Can you work these out from the model? Positions are in its coordinate system, mm. Face numbers are marked on the shaded views. A direction names the side the tool comes from. Coordinates: 2 decimals unless noted, no trailing zeros. Loops run counter-clockwise (first coordinate to the right, second up) from the corner with the lowest first, then second, coordinate; pieces in that order, holes last.
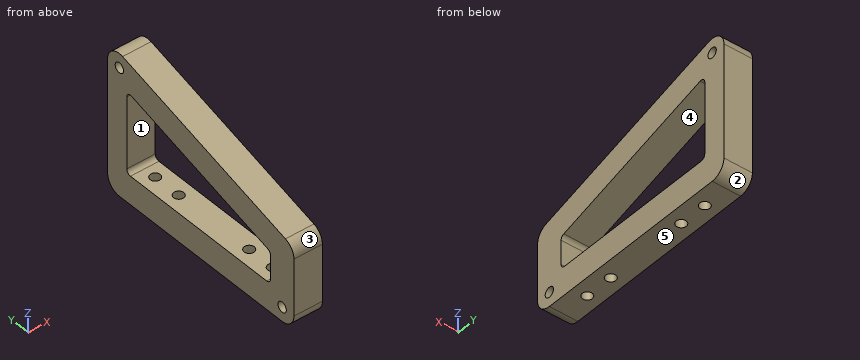
```python
from build123d import *

# Parameters (mm, degrees)
SKETCH1_R           = 2.25
BOSS_EXTRUDE1_DEPTH = 12.7
CUT_EXTRUDE1_REACH  = 117.6
SKETCH3_R           = 2.25
FILLET3_R           = 6.35
FILLET4_R           = 2


with BuildPart() as part:
    # Sketch1 → Boss-Extrude1 (new body)
    with BuildSketch(Plane(origin=(0, 0, 0), x_dir=(0, 0, -1), z_dir=(1, 0, 0))):
        Polygon((6.35, -6.35), (6.35, 94.338181024), (-59.242376653, 94.338181024), (-30.176202444, -6.35), align=None)
        Circle(SKETCH1_R, mode=Mode.SUBTRACT)
        with Locations((-50.8, 87.988181024)):
            Circle(SKETCH1_R, mode=Mode.SUBTRACT)
        Polygon((-6.35, 6.35), (-6.35, 83.988181024), (-43.036009913, 83.988181024), (-20.623797556, 6.35), align=None, mode=Mode.SUBTRACT)
    extrude(amount=BOSS_EXTRUDE1_DEPTH)

    # Sketch3 → Cut-Extrude1 (cut, up to next)
    with BuildSketch(Plane(origin=(0, 0, -6.35), x_dir=(-1, 0, 0), z_dir=(0, 0, -1)), mode=Mode.PRIVATE) as cut_extrude1_sk1:
        with Locations(Location((-6.269939037, 76.2, 0), (0, 0, 90))):
            Circle(SKETCH3_R)
    cut_extrude1_tool1 = extrude(cut_extrude1_sk1.sketch, amount=-CUT_EXTRUDE1_REACH, mode=Mode.PRIVATE) & part.part
    # Sketch3 → Cut-Extrude1 (cut, up to next)
    with BuildSketch(Plane(origin=(0, 0, -6.35), x_dir=(-1, 0, 0), z_dir=(0, 0, -1)), mode=Mode.PRIVATE) as cut_extrude1_sk2:
        with Locations(Location((-6.269939037, 63.5, 0), (0, 0, 90))):
            Circle(SKETCH3_R)
    cut_extrude1_tool2 = extrude(cut_extrude1_sk2.sketch, amount=-CUT_EXTRUDE1_REACH, mode=Mode.PRIVATE) & part.part
    # Sketch3 → Cut-Extrude1 (cut, up to next)
    with BuildSketch(Plane(origin=(0, 0, -6.35), x_dir=(-1, 0, 0), z_dir=(0, 0, -1)), mode=Mode.PRIVATE) as cut_extrude1_sk3:
        with Locations(Location((-6.269939037, 12.7, 0), (0, 0, 90))):
            Circle(SKETCH3_R)
    cut_extrude1_tool3 = extrude(cut_extrude1_sk3.sketch, amount=-CUT_EXTRUDE1_REACH, mode=Mode.PRIVATE) & part.part
    # Sketch3 → Cut-Extrude1 (cut, up to next)
    with BuildSketch(Plane(origin=(0, 0, -6.35), x_dir=(-1, 0, 0), z_dir=(0, 0, -1)), mode=Mode.PRIVATE) as cut_extrude1_sk4:
        with Locations(Location((-6.269939037, 25.4, 0), (0, 0, 90))):
            Circle(SKETCH3_R)
    cut_extrude1_tool4 = extrude(cut_extrude1_sk4.sketch, amount=-CUT_EXTRUDE1_REACH, mode=Mode.PRIVATE) & part.part
    add(cut_extrude1_tool1.solids().sort_by_distance((6.269939, 76.2, -6.35))[0], mode=Mode.SUBTRACT)
    add(cut_extrude1_tool2.solids().sort_by_distance((6.269939, 63.5, -6.35))[0], mode=Mode.SUBTRACT)
    add(cut_extrude1_tool3.solids().sort_by_distance((6.269939, 12.7, -6.35))[0], mode=Mode.SUBTRACT)
    add(cut_extrude1_tool4.solids().sort_by_distance((6.269939, 25.4, -6.35))[0], mode=Mode.SUBTRACT)

    # Fillet3
    fillet3_edges = [part.edges().sort_by_distance(p)[0] for p in [
        (6.35, 94.338181024, 59.242376653),
        (6.35, 94.338181024, -6.35),
        (6.35, -6.35, -6.35),
        (6.35, -6.35, 30.176202444),
    ]]
    fillet(fillet3_edges, radius=FILLET3_R)

    # Fillet4
    fillet4_edges = [part.edges().sort_by_distance(p)[0] for p in [
        (6.35, 83.988181024, 43.036009913),
        (6.35, 6.35, 20.623797556),
        (6.35, 6.35, 6.35),
        (6.35, 83.988181024, 6.35),
    ]]
    fillet(fillet4_edges, radius=FILLET4_R)


solid = part.part
```
Item 1: I'm going to push flat-ended pins straight in: P1, Ø6, axis at y = 87.99, z = 50.8, coming from the -X side; P2, Ø2, axis at x = 9.5, y = 26.5, coming from the +Z side; P3, Ø1.5, axis at x = 10, y = 23.5, coming from the +Z side; P4, Ø4, axis at x = 6.27, y = 76.2, coming from the +Z side. Where does each tip first touch, or does it pass through?
Results are:
P1: stops at x = 0
P2: stops at z = 39.95
P3: stops at z = 39.01
P4: stops at z = 54.58
Item 2: Suppose I cut it at C-C, the plane z = 46.5. Please give me the cut outline in (x, y), plus the area to 3 significant figures.
Results are:
outline: (0, 50.2) - (12.7, 50.2) - (12.7, 94.34) - (0, 94.34) - close
area: 561 mm2
Item 3: On a 3-axis mill with a long thin cutter (end or side, diameter ignored), from which of +Z, -Z, +X, -X, +Y, -Y can I reach the whole of each face in a straight line? I mean the marked faces 1 and 2. Say none if no direction works.
Results are:
face 1: +X, -X
face 2: -Z, +X, -X, +Y
Item 4: We'd pull the mould along Z, two halves only. Please class the marked faces 3, 4 and 5: +Z half, -Z half, draft (parallel to the pull), parting line (faces both ways), or undercut.
Results are:
face 3: +Z half
face 4: undercut
face 5: -Z half
Item 5: I need wall thicknesses on line 1 along X through (y, z) = (63.5, -0.75); line 2 along Y through (x, z) = (1, 14); line 3 along Y through (x, z) = (8.75, 0). Which ranges of each line are inside material? Lowest first, please.
Results are:
line 1: x = 0 to 4.02, 8.52 to 12.7
line 2: y = -6.35 to 6.35, 83.99 to 94.34
line 3: y = -6.35 to -2.25, 2.25 to 94.34
Item 6: Suppose I cut it at A-A, the plane z = 38.5. Please give me the cut outline in (x, y).
Results are:
outline: (0, 22.48) - (12.7, 22.48) - (12.7, 68.27) - (0, 68.27) - close; (0, 83.99) - (12.7, 83.99) - (12.7, 94.34) - (0, 94.34) - close
Item 7: Suppose I cut it at B-B, the plane y = 76.2. Please give me the cut outline in (x, z).
Results are:
outline: (0, -6.35) - (4.02, -6.35) - (4.02, 6.35) - (0, 6.35) - close; (0, 40.79) - (12.7, 40.79) - (12.7, 54.01) - (0, 54.01) - close; (8.52, -6.35) - (12.7, -6.35) - (12.7, 6.35) - (8.52, 6.35) - close
